Autodesk Inventor part; units mm, degrees
ref_plane "YZ Plane" through (0, 0, 0) normal (1, 0, 0) x (0, 1, 0)
ref_plane "XZ Plane" through (0, 0, 0) normal (0, 1, 0) x (-1, 0, 0)
ref_plane "XY Plane" through (0, 0, 0) normal (0, 0, 1) x (1, 0, 0)
sketch "Sketch1" plane through (0, 0, 0) normal (0, 0, 1) x (1, 0, 0)
  line L0 (0, 0) -> (6.223, 0)
  line L1 (0, 0) -> (6.223, 0) construction
  line L2 (6.223, 0) -> (6.223, 38.1)
  line L3 (0, 0) -> (0.762, 0)
  line L4 (0.762, 0) -> (0.762, 8.255)
  line L5 (0.762, 8.255) -> (6.223, 28.6357)
  line L6 (6.223, 28.6357) -> (6.223, 38.1)
  line L7 (0, 0) -> (12.7, 0)
  line L8 (0, -8.9154) -> (0, 53.4924)
  line L9 (6.223, 38.1) -> (12.2033, 44.0803)
  line L10 (6.223, 38.1) -> (14.6805, 38.1) construction
  line L11 (12.2033, 44.0803) -> (12.7, 0)
  line L12 (12.7, 0) -> (12.7, 44.577)
  line L13 (12.7, 44.577) -> (6.223, 38.1)
  dimension "d0" = 6.223
  dimension "d1" = 0
  dimension "d2" = 38.1
  dimension "d3" = 90
  dimension "d4" = 0.762
  dimension "d5" = 8.255
  dimension "d6" = 165
  dimension "d7" = 12.7
  dimension "d18" = 45
revolve "Revolution1" add sketch "Sketch1" angle 360 about axis through (0, -10, 0) along (0, 1, 0)
sketch "Sketch3" plane through (0, 0, 0) normal (0, -1, 0) x (1, 0, 0)
  point P0 (0, 0)
  point P1 (0, 0)
hole "Hole2" at (0, 0, 0) direction (0, 1, 0) diameter 5.3594 depth 6.35
sketch "Sketch4" plane through (0, 0, 0) normal (1, 0, 0) x (0, 1, 0)
  line L0 (0, 12.7) -> (0, -12.7)
  line L1 (0, 12.7) -> (0, 7.9248)
  line L2 (0, 7.9248) -> (12.7, 7.9248)
  line L3 (0, -12.7) -> (0, -7.9248)
  line L4 (0, -7.9248) -> (12.7, -7.9248)
  point P0 (0, 0)
  dimension "d28" = 4.7752
  dimension "d29" = 12.7
  dimension "d30" = 4.7752
  dimension "d31" = 12.7
  dimension "d32" = 90
hole "Hole3" at (0, 12.7, 7.9248) at (0, 12.7, -7.9248) direction (-1, 0, 0) diameter 4.4958 end through all
mirror "Mirror1" about plane through (0, 0, 0) normal (1, 0, 0) of "Hole3"
equation "\"d47\" = 55deg"
equation "\"Sketch5_Pitch\" = 0.90714"
properties part number "catch vertical seal-tighttol-thread"
Verification items for the finished model (mm, model axes). A direction names the side the tool comes from. Round coordinates to 2 decimals unless told otherwise and drop trailing zeros. Write each loop counter-clockwise with the first axis right and the second up, starting at its lowest first coordinate (ties: lowest second). Pieces come first, ordered by that corner, then holes. Notation, with made-up numbers: (38.5, -8.75) -> (50.5, -8.75) arc R23 ccw to (50.5, 9.25) -> close; hole circle Ø2 at (-11.75, 29.25). An arc over 180 degrees is marked (long way). Write each question's results on one line, items separated by ' | '. Start each with the question number.
1. Cross-section at C-C (y = 20.5). Enter the section's corners in (x, z), then the cut area to 3 significant figures.
2. Depth check by flat-ended pin: P1, Ø2, axis at x = -5, y = 20.5, coming from the +Z side; P2, Ø12, axis at x = 6.5, y = 20.5, coming from the -Z side; P3, Ø4.5, axis at x = 0, z = 0, coming from the -Y side. Enter the tip coordinate at first touch or a pass-through.
3. Set-up check for faces 4 (the cylindrical face through (-0.118, 3.219, 2.677)), 5 (the cylindrical face through (-1.349, 33.434, 6.075)), 6 (the cylindrical face through (-0.16, 12.6, -5.68)): record each of +Z, -Z, +X, -X, +Y, -Y from which the full face is reachable in a straight line by a thin tool's end or side.
4. Draft check along Z on faces 1 (the flat face through (1, 6.35, -1)), 2 (the cylindrical face through (12.114, 22.601, -3.815)), 3 (the flat face through (0, 0, -3)). Enter one of: +Z half, -Z half, draft (parallel to the pull), parting line (faces both ways), or undercut.
5. Cross-section at B-B (y = 32). Enter the section's corners in (x, z).
6. Material ranges on probe 1 along Z at (x, y) = (0, 6.8); probe 2 along X at (y, z) = (31, 0); probe 3 along X at (y, z) = (2.75, 0), recorded low to high. Write a range as from..to.
7. Cross-section at A-A (y = 12.7). Enter the section's corners in (x, z), then the cut area to 3 significant figures.
Solutions:
1) outline: circle Ø25.4 at (0, 0); hole circle Ø8.09 at (0, 0) | area: 455 mm2
2) P1: stops at z = 12.05 | P2: stops at z = -12.69 | P3: stops at y = 6.35
3) face 4: -Y | face 5: +Y | face 6: +X, -X
4) face 1: undercut | face 2: parting line | face 3: draft
5) outline: circle Ø25.4 at (0, 0); hole circle Ø12.45 at (0, 0)
6) probe 1: z = -12.7..-0.76, 0.76..12.7 | probe 2: x = -12.7..-6.22, 6.22..12.7 | probe 3: x = -12.7..-2.68, 2.68..12.7
7) outline: (-11.36, -5.68) -> (11.36, -5.68) arc R12.7 ccw to (11.36, 5.68) -> (-11.36, 5.68) arc R12.7 ccw to start; (-7.6, -10.17) arc R12.7 ccw to (7.6, -10.17) -> close; (-7.6, 10.17) -> (7.6, 10.17) arc R12.7 ccw to start; hole circle Ø3.91 at (0, 0) | area: 319 mm2
